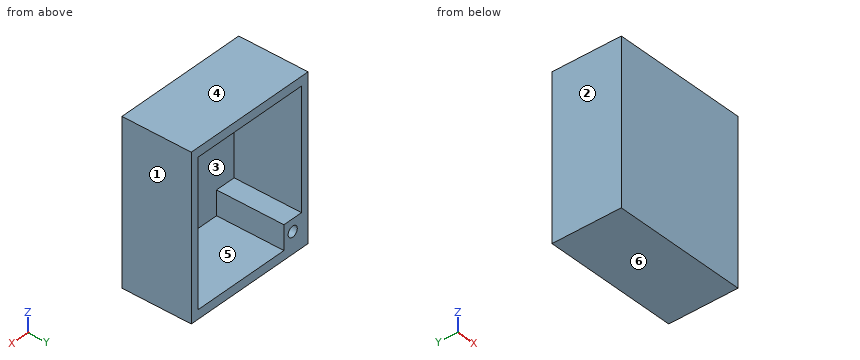
```python
from build123d import *

# Parameters (mm, degrees)
SKETCH_1_W      = 50
SKETCH_1_H      = 60
SKETCH_1_W_2    = 44.384719817
SKETCH_1_H_2    = 53.261663781
SKETCH_1_W_3    = 7.520038949
SKETCH_1_H_3    = 9.02404674
SKETCH_1_R      = 1.953472296
EXTRUDE_1_DEPTH = 25
SKETCH_2_W      = 50
SKETCH_2_H      = 0.716883707
EXTRUDE_2_DEPTH = 60


with BuildPart() as part:
    # Эскиз1 → Бобышка-Вытянуть1 (new body)
    # profile 1 of 2: a face of its own
    with BuildSketch(Plane(origin=(0, 0, 0), x_dir=(1, 0, 0), z_dir=(0, 1, 0))):
        with Locations((25.024105357, 30.007635335)):
            Rectangle(SKETCH_1_W, SKETCH_1_H)
        with Locations((25.024105358, 30.007635335)):
            Rectangle(SKETCH_1_W_2, SKETCH_1_H_2, mode=Mode.SUBTRACT)
    # profile 2 of 2: a face of its own
    with BuildSketch(Plane(origin=(0, 0, 0), x_dir=(1, 0, 0), z_dir=(0, 1, 0))):
        with Locations((6.591764924, 52.126443855)):
            Rectangle(SKETCH_1_W_3, SKETCH_1_H_3)
        with Locations(Location((6.591764924, 52.126443855, 0), (0, 0, 270))):
            Circle(SKETCH_1_R, mode=Mode.SUBTRACT)
    extrude(amount=EXTRUDE_1_DEPTH)

    # Эскиз2 → Бобышка-Вытянуть2 (add)
    with BuildSketch(Plane.XY.offset(-0.007635335)):
        with Locations((25.024105357, -0.358441854)):
            Rectangle(SKETCH_2_W, SKETCH_2_H)
    extrude(amount=-EXTRUDE_2_DEPTH)


solid = part.part
```
For this review, take the finished solid that the model builds, in its own axes (mm). Face numbers are marked on the shaded views. A direction names the side the tool comes from. Coordinates: 2 decimals unless noted, no trailing zeros. Loops run counter-clockwise (first coordinate to the right, second up) from the corner with the lowest first, then second, coordinate; pieces in that order, holes last. Notation, with made-up numbers: (-30, 45.25) -> (17, 45.25) arc R25 ccw to (17, 57.25) -> close; hole circle Ø11 at (29.5, 78.25). An arc over 180 degrees is marked (long way). Return JSON: item names as keys, results as strings. Group by question number.
(1) To check wall thickness, follow L1, parallel to Z at x = 44, y = 6.75; L2, parallel to X at y = 16, z = -17.5; L3, parallel to Z at x = 5.5, y = 1. State the ranges of each line that lie inside material, in increasing order.
(2) Mouldability with a two-part tool opening along X and no side actions: class the marked faces 1, 2, 3 and 4 as pulls with the +X half, pulls with the -X half, needs draft (parallel to the pull), parting line crosses it, or undercut.
(3) Tool access review of the marked faces 5 and 6: name each direction out of +Z, -Z, +X, -X, +Y, -Y from which nothing blocks a thin tool from reaching the whole face with its end or side.
(4) Consider section A-A, the plane z = -49.5. Give the boundary of the cut face in (x, y), plus the area to 3 significant figures.
(5) Consider section B-B, the plane y = 10.75. Give the boundary of the cut face in (x, z), plus the area to 3 significant figures.
(6) Consider section C-C, the plane z = -36. Give the boundary of the cut face in (x, y).
(7) For pin 1 Ø2 at (x, z) = (6.5, -51.5) entering from +Y, flat-tipped, find the tip position at first contact; note if it passes through.
Results below:
{
 "1": {"L1": "z = -60.01 to -56.64, -3.38 to -0.01", "L2": "x = 0.02 to 2.83, 47.22 to 50.02", "L3": "z = -60.01 to -53.75, -50.51 to -47.61, -3.38 to -0.01"},
 "2": {"face 1": "pulls with the +X half", "face 2": "pulls with the -X half", "face 3": "undercut", "face 4": "needs draft"},
 "3": {"face 5": "+Y", "face 6": "-Z, +X, -X, +Y, -Y"},
 "4": {"outline": "(0.02, -0.72) -> (50.02, -0.72) -> (50.02, 25) -> (47.22, 25) -> (47.22, 0) -> (10.35, 0) -> (10.35, 25) -> (0.02, 25) -> close", "area": "364 mm2"},
 "5": {"outline": "(0.02, -60.01) -> (50.02, -60.01) -> (50.02, -0.01) -> (0.02, -0.01) -> close; hole (2.83, -47.61) -> (10.35, -47.61) -> (10.35, -56.64) -> (47.22, -56.64) -> (47.22, -3.38) -> (2.83, -3.38) -> close; hole circle Ø3.91 at (6.59, -52.13)", "area": "692 mm2"},
 "6": {"outline": "(0.02, -0.72) -> (50.02, -0.72) -> (50.02, 25) -> (47.22, 25) -> (47.22, 0) -> (2.83, 0) -> (2.83, 25) -> (0.02, 25) -> close"},
 "7": {"pin 1": "stops at y = 0"}
}
